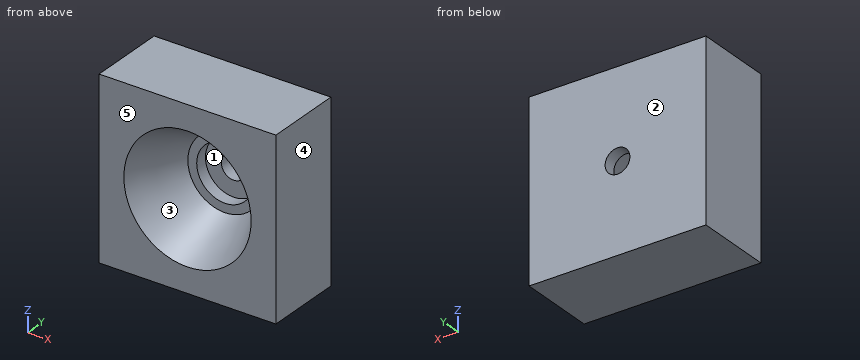
from build123d import *

# Parameters (mm, degrees)
BOSS_EXTRUDE1_DEPTH      = 11
BOSS_EXTRUDE1_DEPTH_BACK = 11
SKETCH1_W                = 50
SKETCH1_H                = 50


with BuildPart() as part:
    # Sketch1 → Boss-Extrude1 (new, two sides: drawn at the far end of the back side and taken through both)
    with BuildSketch(Plane(origin=(0, 0, 0), x_dir=(1, 0, 0), z_dir=(0, 1, 0)).offset(-BOSS_EXTRUDE1_DEPTH_BACK)):
        Rectangle(SKETCH1_W, SKETCH1_H)
    extrude(amount=BOSS_EXTRUDE1_DEPTH + BOSS_EXTRUDE1_DEPTH_BACK)

    # Sketch2 → Cut-Revolve1 (revolve, cut)
    with BuildSketch(Plane.XY):
        Polygon((-3.5, 7.5), (-3.5, 11), (0, 11), (0, -11), (-18, -11), (-10.5, 4), (-8, 4), (-8, 7.5), align=None)
    revolve(axis=Axis((0, 11, 0), (0, -1, 0)), mode=Mode.SUBTRACT)


solid = part.part
Source: CAD feature listing. Evaluate the final solid. Frame: model axes, mm. Face numbers are marked on the shaded views. A direction names the side the tool comes from. Round coordinates to 2 decimals unless told otherwise and drop trailing zeros. Loops run counter-clockwise (first coordinate to the right, second up) from the corner with the lowest first, then second, coordinate; pieces in that order, holes last. Notation, with made-up numbers: M 32.5,-39.5 L 38.5,-39.5 A21 ccw 38.5,-23.5 Z; hole C 53,-17 d1. An arc over 180 degrees is marked long. Answer as CSV lines item,"result".
Q1. Cut plane B-B (y = 6.25). Return the cut outline in (x, z), plus the area to 3 significant figures.
Verdict:
outline,"M -25,-25 L 25,-25 L 25,25 L -25,25 Z; hole C 0,0 d16"
area,"2,300 mm^2"
Q2. Cut plane A-A (x = 0). Return the cut outline in (y, z), plus the area to 3 significant figures.
Verdict:
outline,"M -11,-25 L 11,-25 L 11,-3.5 L 7.5,-3.5 L 7.5,-8 L 4,-8 L 4,-10.5 L -11,-18 Z; M -11,18 L 4,10.5 L 4,8 L 7.5,8 L 7.5,3.5 L 11,3.5 L 11,25 L -11,25 Z"
area,"592 mm^2"
Q3. Pull-direction query (X, two-part tool) for the marked faces 3, 4 and 5; classes: +X half, -X half, draft (parallel to the pull), parting line (faces both ways), or undercut.
Verdict:
face 3,"undercut"
face 4,"+X half"
face 5,"draft"
Q4. Line query: line 1 along X through (y, z) = (6.65, 0); line 2 along X through (y, z) = (9.95, 0). Output: solid intervals per line, ascending.
Verdict:
line 1,"x = -25 to -8, 8 to 25"
line 2,"x = -25 to -3.5, 3.5 to 25"
Q5. Cut plane C-C (z = 0). Return the cut outline in (x, y).
Verdict:
outline,"M -25,-11 L -18,-11 L -10.5,4 L -8,4 L -8,7.5 L -3.5,7.5 L -3.5,11 L -25,11 Z; M 3.5,7.5 L 8,7.5 L 8,4 L 10.5,4 L 18,-11 L 25,-11 L 25,11 L 3.5,11 Z"
Q6. Cut plane D-D (y = -9.5). Return the cut outline in (x, z).
Verdict:
outline,"M -25,-25 L 25,-25 L 25,25 L -25,25 Z; hole C 0,0 d34.5"
Q7. Reachability of the marked faces 1 and 2 from +Z, -Z, +X, -X, +Y, -Y: full face, straight path, thin tool, end or side. Return the list, or none.
Verdict:
face 1,"-Y"
face 2,"+Z, -Z, +X, -X, +Y"
Q8. Contact query for flat-ended pins moving along their axis: pin 1 (17.5 mm diameter, centred on x = 3, z = 0.5, fed in from -Y); pin 2 (1.5 mm diameter, centred on x = -5.5, z = -10, fed in from -Y); pin 3 (10.5 mm diameter, centred on x = 4, z = 2.5, fed in from -Y). Output: stop coordinate, or through.
Verdict:
pin 1,"stops at y = 1.42"
pin 2,"stops at y = 0.67"
pin 3,"stops at y = 4"
